Geometry check sheet. Reference: the model listing, model coordinates, mm. A direction names the side the tool comes from. Give positions to 0.01 mm unless a question says otherwise; leave off trailing zeros. Order: outer loops, then holes, each group sorted by start corner. A loop starts at its lowest first (then second) coordinate and runs counter-clockwise, first axis right, second up.
Solid Edge part; units mm, degrees
sketch "Sketch1" plane through (-117, 0, 0) normal (1, 0, 0) x (0, 1, 0)
  line L0 (80.9905, 27.2958) -> (116.9905, 27.2958)
  line L1 (116.9905, 27.2958) -> (116.9905, 8)
  line L2 (80.9905, 8) -> (116.9905, 8)
  line L3 (80.9905, 27.2958) -> (80.9905, 8)
extrude "Protrusion1" add sketch "Sketch1" along normal blind 42.5
fillet "Round_2" radius 7 1 edges at (-95.75, 116.9905, 8)
sketch "Sketch2" plane through (-74.5, 98.9905, 18.3979) normal (1, 0, 0) x (0, 1, 0)
  line L0 (-11.25, 9.3979) -> (-11.25, -10.3979)
  line L1 (-11.25, -10.3979) -> (1.25, -10.3979)
  line L2 (1.25, -10.3979) -> (1.25, 9.3979)
  line L3 (-11.25, 9.3979) -> (1.25, 9.3979)
extrude "ExtrudedCutout_7" cut sketch "Sketch2" against normal blind 23.2
sketch "Sketch3" plane through (-74.5, 98.9905, 18.3979) normal (1, 0, 0) x (0, 1, 0)
  circle A0 centre (-14.7, 2.8979) radius 1.2
  circle A1 centre (4.7, 2.8979) radius 1.2
extrude "ExtrudedCutout_8" cut sketch "Sketch3" against normal blind 10
Q1. Cross-section at A-A, the plane x = -96. Record the boundary of the cut face in (y, z).
Q2. Cross-section at D-D, the plane x = -109.5. Record the boundary of the cut face in (y, z).
Q3. Release check for a two-part mould opening along Z. For faces 1 (the face through (-84.5, 84, 21)), 2 (the face through (-79.43, 104.336, 22.308)), 3 (the face through (-95.45, 114.89, 10)), 4 (the face through (-96, 116.99, 21)) record: pulls with the +Z half, pulls with the -Z half, needs draft (parallel to the pull), parting line crosses it, or undercut.
Q4. Access from +Z, -Z, +X, -X, +Y, -Y to the whole of each face (thin tool, end or side, straight path). Record for faces 5 (the face through (-97.7, 94, 18)), 6 (the face through (-84.5, 104, 21)), 7 (the face through (-74.5, 108, 18)).
Q5. Thickness scan on L1, parallel to Y at x = -82, z = 15; L2, parallel to X at y = 91.5, z = 19; L3, parallel to Y at x = -85.5, z = 10. Record the ranges inside material, lowest first.
Q6. Gauge pin test, flat ends, axial feed: P1, Ø6, axis at y = 92, z = 17, coming from the +X side; P2, Ø1.2, axis at y = 104, z = 21.5, coming from the +X side. Record the tip position at first contact, or that the pin passes through.
Q7. Cross-section at C-C, the plane z = 25.75. Record the boundary of the cut face in (x, y), and give its area (3 significant figures).
Q8. Cross-section at B-B, the plane x = -78. Record the boundary of the cut face in (y, z).
Answers follow:
1. outline: (80.99, 8) - (87.74, 8) - (87.74, 27.3) - (80.99, 27.3) - close; (100.24, 8) - (109.99, 8) arc R7 ccw to (116.99, 15) - (116.99, 27.3) - (100.24, 27.3) - close
2. outline: (80.99, 8) - (109.99, 8) arc R7 ccw to (116.99, 15) - (116.99, 27.3) - (80.99, 27.3) - close
3. face 1: undercut
3. face 2: undercut
3. face 3: pulls with the -Z half
3. face 4: needs draft
4. face 5: +Z, -Z, +X
4. face 6: +X
4. face 7: +Z, -Z, +X, +Y, -Y
5. L1: y = 80.99 to 87.74, 100.24 to 116.99
5. L2: x = -117 to -97.7
5. L3: y = 80.99 to 87.74, 100.24 to 114.89
6. P1: stops at x = -97.7
6. P2: stops at x = -84.5
7. outline: (-117, 80.99) - (-74.5, 80.99) - (-74.5, 87.74) - (-97.7, 87.74) - (-97.7, 100.24) - (-74.5, 100.24) - (-74.5, 116.99) - (-117, 116.99) - close
7. area: 1,240 mm2
8. outline: (80.99, 8) - (87.74, 8) - (87.74, 27.3) - (80.99, 27.3) - close; (100.24, 8) - (109.99, 8) arc R7 ccw to (116.99, 15) - (116.99, 27.3) - (100.24, 27.3) - close; hole circle Ø2.4 at (84.29, 21.3); hole circle Ø2.4 at (103.69, 21.3)
